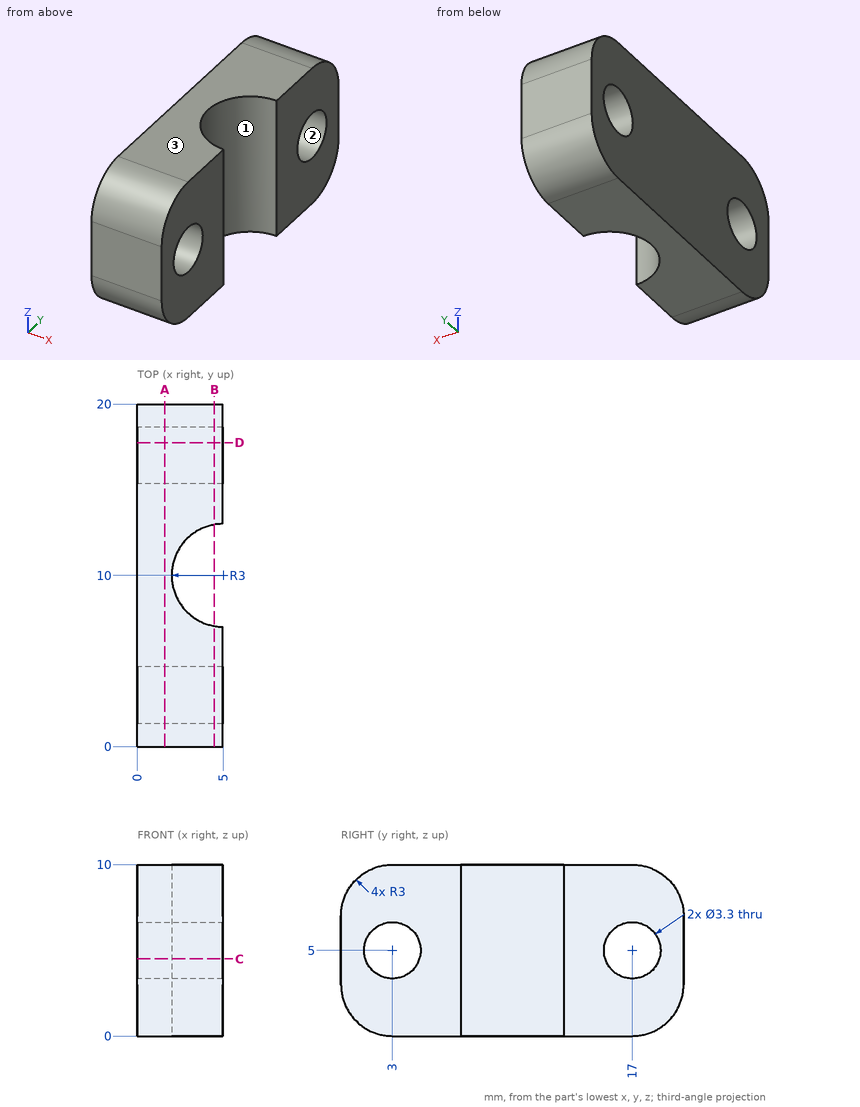
Can you work these out from the drawing? Everything is in mm from the part's minimum corner. Give positions to 0.01 mm unless a question says otherwise; leave off trailing zeros. Write each loop counter-clockwise with the first axis right and the second up, starting at its lowest first coordinate (ties: lowest second). Pieces come first, ordered by that corner, then holes. Notation, with made-up numbers: (88.25, 35.5) -> (135.25, 35.5) arc R21 ccw to (135.25, 43.5) -> close; hole circle Ø5 at (-24, -38). An arc over 180 degrees is marked (long way). Write each question's results on one line, items separated by ' | '. Start each with the question number.
Q1. I need wall thicknesses on probe 1 along Y at (x, z) = (1.1, 5); probe 2 along Y at (x, z) = (2.5, 5); probe 3 along Y at (x, z) = (3.85, 5.5). Which ranges of each line are inside material? Lowest first, please.
Q2. Suppose I cut it at D-D, the plane y = 17.75. List the corners of the cut face in (x, z) for me, and give its area (3 significant figures).
Q3. Suppose I cut it at C-C, the plane z = 4.5. List the corners of the cut face in (x, y) for me.
Q4. We'd pull the mould along Z, two halves only. Please class the marked faces 1, 2 and 3: +Z half, -Z half, draft (parallel to the pull), parting line (faces both ways), or undercut.
Q5. Suppose I cut it at A-A, the plane x = 1.6. List the corners of the cut face in (y, z) for me, and give its area (3 significant figures).
Q6. Suppose I cut it at B-B, the plane x = 4.5. List the corners of the cut face in (y, z) for me.
Outcome:
1) probe 1: 0 to 1.35, 4.65 to 15.35, 18.65 to 20 | probe 2: 0 to 1.35, 4.65 to 8.34, 11.66 to 15.35, 18.65 to 20 | probe 3: 0 to 1.43, 4.57 to 7.23, 12.77 to 15.43, 18.57 to 20
2) outline: (0, 0.1) -> (5, 0.1) -> (5, 3.53) -> (0, 3.53) -> close; (0, 6.47) -> (5, 6.47) -> (5, 9.9) -> (0, 9.9) -> close | area: 34.4 mm2
3) outline: (0, 0) -> (5, 0) -> (5, 1.43) -> (0, 1.43) -> close; (0, 4.57) -> (5, 4.57) -> (5, 7) arc R3 cw to (5, 13) -> (5, 15.43) -> (0, 15.43) -> close; (0, 18.57) -> (5, 18.57) -> (5, 20) -> (0, 20) -> close
4) face 1: draft | face 2: undercut | face 3: +Z half
5) outline: (0, 3) arc R3 ccw to (3, 0) -> (17, 0) arc R3 ccw to (20, 3) -> (20, 7) arc R3 ccw to (17, 10) -> (3, 10) arc R3 ccw to (0, 7) -> close; hole circle Ø3.3 at (3, 5); hole circle Ø3.3 at (17, 5) | area: 175 mm2
6) outline: (0, 3) arc R3 ccw to (3, 0) -> (7.04, 0) -> (7.04, 10) -> (3, 10) arc R3 ccw to (0, 7) -> close; (12.96, 0) -> (17, 0) arc R3 ccw to (20, 3) -> (20, 7) arc R3 ccw to (17, 10) -> (12.96, 10) -> close; hole circle Ø3.3 at (3, 5); hole circle Ø3.3 at (17, 5)
